Build history of the part. All positions in model axes, mm. A direction names the side the tool comes from. Give positions to 0.01 mm unless a question says otherwise; leave off trailing zeros. Order: outer loops, then holes, each group sorted by start corner. A loop starts at its lowest first (then second) coordinate and runs counter-clockwise, first axis right, second up. Notation, with made-up numbers: M 61,51.25 L 105,51.25 A32 cw 105,87.25 Z; hole C 62.25,-16.75 d8. An arc over 180 degrees is marked long. Use CSV: the item, a comma, the result in double quotes. Start each with the question number.
Item 1: Pin check, flat tips, straight feed: P1, Ø14.5, axis at x = 16, y = -9, coming from the +Z side; P2, Ø5, axis at y = 13.5, z = 9.5, coming from the +X side; P3, Ø8, axis at x = -33, z = 14, coming from the +Y side. Stop position of each tip, or through.
Item 2: Band-saw the part on D-D on z = 23. Write the cut outline in (x, y), plus the area to 3 significant figures.
Item 3: Two-plate mould, pull along Y, no slides. Class faces 3 (the cylindrical face through (-38.505, -10.648, 14.86)), 4 (the flat face through (-28, 4, 5)), 5 (the flat face through (-10, 5, 25)): pulls with the +Y half, pulls with the -Y half, needs draft (parallel to the pull), parting line crosses it, or undercut.
Item 4: Band-saw the part on B-B on x = 18.5. Write the cut outline in (y, z).
Item 5: Band-saw the part on C-C on y = 0. Write the cut outline in (x, z).
Item 6: Wall check: line 1 along Y through (x, z) = (18.5, 3.4); line 2 along Y through (x, z) = (-24, 13.25); line 3 along Z through (x, y) = (26, -4.5). Give the ranges that are in metal, low to high.
Item 7: Which spindle directions (+Z, -Z, +X, -X, +Y, -Y) get a long thin tool onto all of the face, cutting with end or side? Do faces 1 (the cylindrical face through (-39.6, 0.7, 15.1)), 2 (the flat face through (35.895, 20.549, 2.535)). Say none if no direction does.
Item 8: Band-saw the part on A-A on z = 3.5. Write the cut outline in (x, y).
from build123d import *

# Parameters (mm, degrees)
BOSS_EXTRUDE2_DEPTH = 5
SKETCH2_R           = 2
CUT_EXTRUDE1_DEPTH  = 50.932454376
SKETCH3_R           = 5
CUT_EXTRUDE2_DEPTH  = 5
CUT_EXTRUDE5_DEPTH  = 50.932454376
SKETCH10_R          = 17.5
BOSS_EXTRUDE5_DEPTH = 20
SKETCH11_R          = 15
CUT_EXTRUDE6_DEPTH  = 20


with BuildPart() as part:
    # Sketch1 → Boss-Extrude2 (new body)
    with BuildSketch(Plane.XY):
        with BuildLine():
            Line((-19.5, 24), (43.5, 24))
            Line((43.5, 24), (43.5, -24))
            Line((43.5, -24), (-19.5, -24))
            ThreePointArc((-19.5, -24), (-43.5, 0), (-19.5, 24))
        make_face()
    extrude(amount=BOSS_EXTRUDE2_DEPTH)

    # Sketch2 → Cut-Extrude1 (cut, through all)
    with BuildSketch(Plane.XY.offset(5)):
        with Locations((33.5, 0)):
            Circle(SKETCH2_R)
        with Locations((18.5, 0)):
            Circle(SKETCH2_R)
    extrude(amount=-CUT_EXTRUDE1_DEPTH, mode=Mode.SUBTRACT)

    # Sketch3 → Cut-Extrude2 (cut)
    with BuildSketch(Plane.XY.offset(5)):
        with Locations((-24.61729874, 0)):
            Circle(SKETCH3_R)
    extrude(amount=-CUT_EXTRUDE2_DEPTH, mode=Mode.SUBTRACT)

    # Sketch9 → Cut-Extrude5 (cut, through all)
    with BuildSketch(Plane.XY.offset(5)):
        Polygon((28.5, 24), (43.5, 17), (43.5, 24), align=None)
        Polygon((43.5, -17), (28.5, -24), (43.5, -24), align=None)
    extrude(amount=-CUT_EXTRUDE5_DEPTH, mode=Mode.SUBTRACT)

    # Sketch10 → Boss-Extrude5 (add)
    with BuildSketch(Plane.XY.offset(5)):
        with Locations((-24.61729874, 0)):
            Circle(SKETCH10_R)
    extrude(amount=BOSS_EXTRUDE5_DEPTH)

    # Sketch11 → Cut-Extrude6 (cut)
    with BuildSketch(Plane.XY.offset(25)):
        with Locations((-24.61729874, 0)):
            Circle(SKETCH11_R)
    extrude(amount=-CUT_EXTRUDE6_DEPTH, mode=Mode.SUBTRACT)


solid = part.part
Model answer:
1,P1,"stops at z = 5"
1,P2,"stops at x = -11.01"
1,P3,"stops at y = 16.94"
2,outline,"C -24.62,0 d35; hole C -24.62,0 d30"
2,area,"255 mm^2"
3,face 3,"parting line crosses it"
3,face 4,"undercut"
3,face 5,"needs draft"
4,outline,"M -24,0 L -2,0 L -2,5 L -24,5 Z; M 2,0 L 24,0 L 24,5 L 2,5 Z"
5,outline,"M -43.5,0 L -29.62,0 L -29.62,5 L -39.62,5 L -39.62,25 L -42.12,25 L -42.12,5 L -43.5,5 Z; M -19.62,0 L 16.5,0 L 16.5,5 L -7.12,5 L -7.12,25 L -9.62,25 L -9.62,5 L -19.62,5 Z; M 20.5,0 L 31.5,0 L 31.5,5 L 20.5,5 Z; M 35.5,0 L 43.5,0 L 43.5,5 L 35.5,5 Z"
6,line 1,"y = -24 to -2, 2 to 24"
6,line 2,"y = -17.49 to -14.99, 14.99 to 17.49"
6,line 3,"z = 0 to 5"
7,face 1,"+Z"
7,face 2,"+Z, -Z, +X, +Y"
8,outline,"M -19.5,-24 L 28.5,-24 L 43.5,-17 L 43.5,17 L 28.5,24 L -19.5,24 A24 ccw Z; hole C -24.62,0 d10; hole C 18.5,0 d4; hole C 33.5,0 d4"
